Input: part model. Units: mm. Frame: model coordinates. A direction names the side the tool comes from. Coordinates: 2 decimals unless noted, no trailing zeros. Loops run counter-clockwise (first coordinate to the right, second up) from the corner with the lowest first, then second, coordinate; pieces in that order, holes last.
Item 1: Section D-D on x = 2.25. Return loops of the section in (y, z).
Item 2: Pull-direction query (X, two-part tool) for faces 3 (the flat face through (12, 24, -3)), 4 (the cylindrical face through (5, 39, -1)), 5 (the flat face through (0, 17.4, -0.4)); classes: released by +X, released by -X, zero draft, split by the parting line, or undercut.
Item 3: Section C-C on y = 41. Return loops of the section in (x, z), and give its area (3 significant figures).
Item 4: Ray query, line 1 along X through (y, z) = (1, 6); line 2 along Z through (x, y) = (9.75, 41.5); line 3 along Y through (x, z) = (9.75, 3.5). Return the intervals inside material, ascending.
Item 5: Contact query for flat-ended pins moving along their axis: P1, Ø8, axis at x = 9.5, y = 26.5, coming from the +Z side; P2, Ø6.5, axis at x = 20, y = 41, coming from the -Z side; P3, Ø2, axis at x = 15, z = 7.5, coming from the +Y side. Output: stop coordinate, or through.
Item 6: Section B-B on z = 6. Return loops of the section in (x, y), and give its area (3 significant figures).
Item 7: Reachability of faces 1 (the cylindrical face through (12.68, 0.86, -2.1)), 2 (the flat face through (12, 3, 6)) from +Z, -Z, +X, -X, +Y, -Y: full face, straight path, thin tool, end or side. Return the list, or none.
Item 8: Section A-A on x = 20. Return loops of the section in (y, z), and give its area (3 significant figures).
```python
from build123d import *

# Parameters (mm, degrees)
SKETCH1_W           = 25
SKETCH1_H           = 45
SKETCH1_R           = 2
BOSS_EXTRUDE1_DEPTH = 3
BOSS_EXTRUDE2_START = -3
SKETCH1_3_W         = 25
SKETCH1_3_H         = 3
BOSS_EXTRUDE2_DEPTH = 13
FILLET1_R           = 3
SKETCH2_R           = 2
CUT_EXTRUDE1_DEPTH  = 46


with BuildPart() as part:
    # Sketch1 → Boss-Extrude1 (new body)
    with BuildSketch(Plane.XY):
        with Locations((12.5, 22.5)):
            Rectangle(SKETCH1_W, SKETCH1_H)
        with Locations((20, 41)):
            Circle(SKETCH1_R, mode=Mode.SUBTRACT)
        with Locations((5, 41)):
            Circle(SKETCH1_R, mode=Mode.SUBTRACT)
    extrude(amount=-BOSS_EXTRUDE1_DEPTH)

    # Sketch1<3> → Boss-Extrude2 (add)
    with BuildSketch(Plane.XY.offset(BOSS_EXTRUDE2_START)):
        with Locations((12.5, 1.5)):
            Rectangle(SKETCH1_3_W, SKETCH1_3_H)
    extrude(amount=BOSS_EXTRUDE2_DEPTH)

    # Fillet1
    fillet1_edges = [part.edges().sort_by_distance(p)[0] for p in [
        (12.5, 3, 0),
        (12.5, 0, -3),
    ]]
    fillet(fillet1_edges, radius=FILLET1_R)

    # Sketch2 → Cut-Extrude1 (cut, through all)
    with BuildSketch(Plane(origin=(0, 0, 0), x_dir=(-1, 0, 0), z_dir=(0, -1, 0))):
        with Locations((-5, -6)):
            Circle(SKETCH2_R)
        with Locations((-20, -6)):
            Circle(SKETCH2_R)
    extrude(amount=-CUT_EXTRUDE1_DEPTH, mode=Mode.SUBTRACT)


solid = part.part
```
Results found:
1. outline: (0, 0) arc R3 ccw to (3, -3) - (45, -3) - (45, 0) - (6, 0) arc R3 cw to (3, 3) - (3, 10) - (0, 10) - close
2. face 3: zero draft
2. face 4: undercut
2. face 5: released by -X
3. outline: (0, -3) - (3, -3) - (3, 0) - (0, 0) - close; (7, -3) - (18, -3) - (18, 0) - (7, 0) - close; (22, -3) - (25, -3) - (25, 0) - (22, 0) - close
3. area: 51.0 mm2
4. line 1: x = 0 to 3, 7 to 18, 22 to 25
4. line 2: z = -3 to 0
4. line 3: y = 0 to 3
5. P1: stops at z = 0
5. P2: stops at z = -3
5. P3: stops at y = 3
6. outline: (0, 0) - (3, 0) - (3, 3) - (0, 3) - close; (7, 0) - (18, 0) - (18, 3) - (7, 3) - close; (22, 0) - (25, 0) - (25, 3) - (22, 3) - close
6. area: 51.0 mm2
7. face 1: -Z, +X, -X, -Y
7. face 2: +Z, +X, -X, +Y
8. outline: (0, 0) arc R3 ccw to (3, -3) - (39, -3) - (39, 0) - (6, 0) arc R3 cw to (3, 3) - (3, 4) - (0, 4) - close; (0, 8) - (3, 8) - (3, 10) - (0, 10) - close; (43, -3) - (45, -3) - (45, 0) - (43, 0) - close
8. area: 141 mm2
